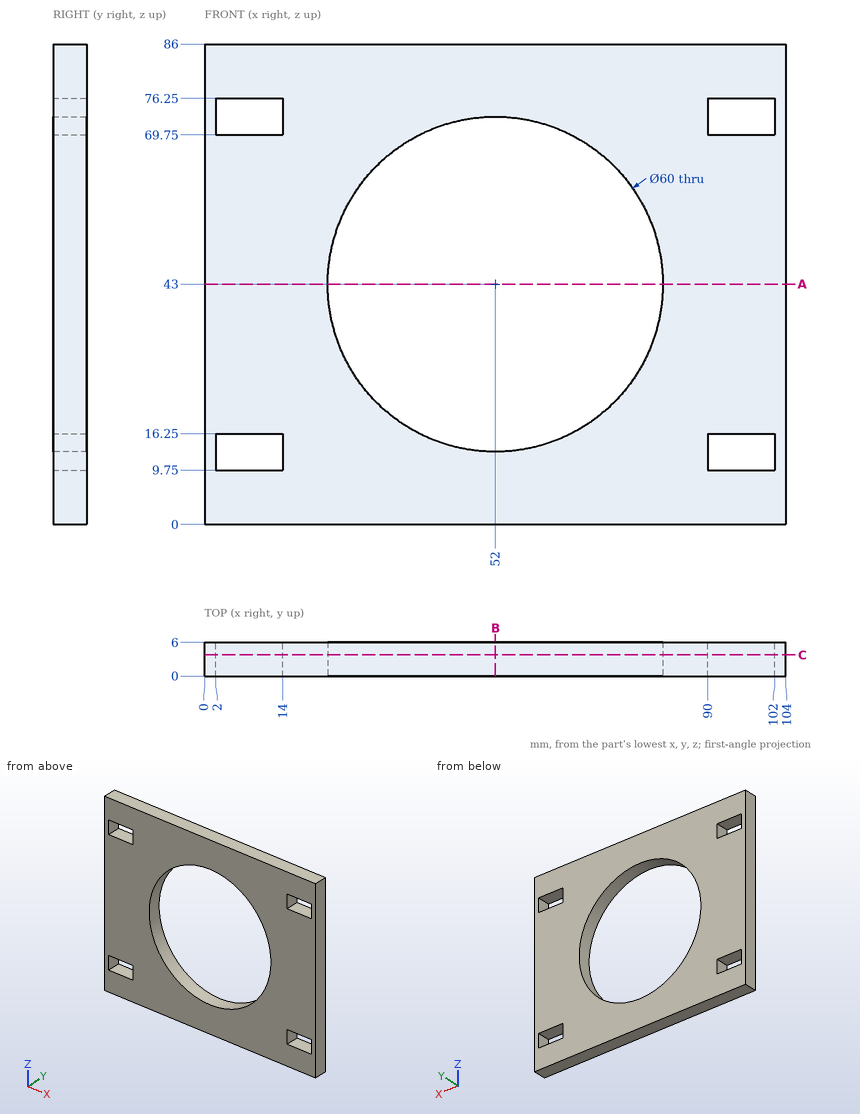
Part print with two shaded views. Sizes in mm from the minimum x, y, z corner. Coordinates: 2 decimals unless noted, no trailing zeros. Write each loop counter-clockwise with the first axis right and the second up, starting at its lowest first coordinate (ties: lowest second). Pieces come first, ordered by that corner, then holes. Notation, with made-up numbers: (38, 29.25) - (83, 29.25) arc R5 ccw to (83, 34.25) - close; hole circle Ø4 at (51, 36.25). An arc over 180 degrees is marked (long way). Use a Markdown table: item, result. Add a question column.
Item 1: Band-saw the part on B-B, the plane x = 52. Write the cut outline in (y, z).
Item 2: Band-saw the part on A-A, the plane z = 43. Write the cut outline in (x, y), and give its area (3 significant figures).
Item 3: Drill centre lines: line 1 along X through (y, z) = (1.45, 75.5); line 2 along X through (y, z) = (4.3, 43); line 3 along X through (y, z) = (5.1, 70.5). Where is each one in solid material? Low to high.
Item 4: Band-saw the part on C-C, the plane y = 3.8. Write the cut outline in (x, z).
A:
| question | item | result |
|---|---|---|
| 1 | outline | (0, 0) - (6, 0) - (6, 13) - (0, 13) - close; (0, 73) - (6, 73) - (6, 86) - (0, 86) - close |
| 2 | outline | (0, 0) - (22, 0) - (22, 6) - (0, 6) - close; (82, 0) - (104, 0) - (104, 6) - (82, 6) - close |
| 2 | area | 264 mm² |
| 3 | line 1 | x = 0 to 2, 14 to 90, 102 to 104 |
| 3 | line 2 | x = 0 to 22, 82 to 104 |
| 3 | line 3 | x = 0 to 2, 14 to 40.01, 63.99 to 90, 102 to 104 |
| 4 | outline | (0, 0) - (104, 0) - (104, 86) - (0, 86) - close; hole (2, 9.75) - (14, 9.75) - (14, 16.25) - (2, 16.25) - close; hole (2, 69.75) - (14, 69.75) - (14, 76.25) - (2, 76.25) - close; hole circle Ø60 at (52, 43); hole (90, 9.75) - (102, 9.75) - (102, 16.25) - (90, 16.25) - close; hole (90, 69.75) - (102, 69.75) - (102, 76.25) - (90, 76.25) - close |
